Check sheet for the modelled part. Datum: model origin and axes. Units: mm. A direction names the side the tool comes from. Give positions to 0.01 mm unless a question says otherwise; leave off trailing zeros. Order: outer loops, then holes, each group sorted by start corner. A loop starts at its lowest first (then second) coordinate and runs counter-clockwise, first axis right, second up. Notation, with made-up numbers: (85.5, 55) -> (102.5, 55) arc R25 ccw to (102.5, 87) -> close; hole circle Ø8 at (76.5, 62). An arc over 180 degrees is marked (long way). Write each question's results on one line, items separated by ' | '.
from build123d import *

# Parameters (mm, degrees)
EXTRUDE1_DEPTH      = 2.794
CUT_EXTRUDE1_DEPTH  = 6.588
SHELL2_T            = 1.016
BOSS_EXTRUDE1_DEPTH = 5.08
BOSS_EXTRUDE2_DEPTH = 0.381


with BuildPart() as part:
    # Sketch1 → Extrude1 (new body, symmetric)
    with BuildSketch(Plane.XY):
        with BuildLine():
            Line((-83.497972353, 1.642657809), (-75.199494217, 5.08))
            Line((-75.199494217, 5.08), (75.199494217, 5.08))
            Line((75.199494217, 5.08), (83.497972353, 1.642657809))
            ThreePointArc((83.497972353, 1.642657809), (84.595561211, 0), (83.497972353, -1.642657809))
            Line((83.497972353, -1.642657809), (75.199494217, -5.08))
            Line((75.199494217, -5.08), (-75.199494217, -5.08))
            Line((-75.199494217, -5.08), (-83.497972353, -1.642657809))
            ThreePointArc((-83.497972353, -1.642657809), (-84.595561211, 0), (-83.497972353, 1.642657809))
        make_face()
    extrude(amount=EXTRUDE1_DEPTH, both=True)

    # Sketch7 → Cut-Extrude1 (cut, through all)
    with BuildSketch(Plane.XY.offset(-2.794)):
        with BuildLine():
            Line((-69.101561211, -1.905), (-68.593561211, -1.905))
            ThreePointArc((-68.593561211, -1.905), (-66.688561211, 0), (-68.593561211, 1.905))
            Line((-68.593561211, 1.905), (-69.101561211, 1.905))
            ThreePointArc((-69.101561211, 1.905), (-71.006561211, 0), (-69.101561211, -1.905))
        make_face()
        with BuildLine():
            Line((69.101561211, -1.905), (68.593561211, -1.905))
            ThreePointArc((68.593561211, -1.905), (66.688561211, 0), (68.593561211, 1.905))
            Line((68.593561211, 1.905), (69.101561211, 1.905))
            ThreePointArc((69.101561211, 1.905), (71.006561211, 0), (69.101561211, -1.905))
        make_face()
    extrude(amount=CUT_EXTRUDE1_DEPTH, mode=Mode.SUBTRACT)

    # Shell2 (no face opened: a closed hollow body)
    add(offset(amount=-SHELL2_T, mode=Mode.PRIVATE), mode=Mode.SUBTRACT)

    # Sketch16 → Boss-Extrude1 (add)
    with BuildSketch(Plane.XY):
        with BuildLine():
            Line((-68.593561211, 3.175), (-69.101561211, 3.175))
            ThreePointArc((-69.101561211, 3.175), (-72.276561211, 0), (-69.101561211, -3.175))
            Line((-69.101561211, -3.175), (-68.593561211, -3.175))
            ThreePointArc((-68.593561211, -3.175), (-65.418561211, 0), (-68.593561211, 3.175))
        make_face()
        with BuildLine():
            Line((-68.593561211, 1.905), (-69.101561211, 1.905))
            ThreePointArc((-69.101561211, 1.905), (-71.006561211, 0), (-69.101561211, -1.905))
            Line((-69.101561211, -1.905), (-68.593561211, -1.905))
            ThreePointArc((-68.593561211, -1.905), (-66.688561211, 0), (-68.593561211, 1.905))
        make_face(mode=Mode.SUBTRACT)
        with BuildLine():
            Line((69.101561211, -3.175), (68.593561211, -3.175))
            ThreePointArc((68.593561211, -3.175), (65.418561211, 0), (68.593561211, 3.175))
            Line((68.593561211, 3.175), (69.101561211, 3.175))
            ThreePointArc((69.101561211, 3.175), (72.276561211, 0), (69.101561211, -3.175))
        make_face()
        with BuildLine():
            Line((69.101561211, -1.905), (68.593561211, -1.905))
            ThreePointArc((68.593561211, -1.905), (66.688561211, 0), (68.593561211, 1.905))
            Line((68.593561211, 1.905), (69.101561211, 1.905))
            ThreePointArc((69.101561211, 1.905), (71.006561211, 0), (69.101561211, -1.905))
        make_face(mode=Mode.SUBTRACT)
    extrude(amount=BOSS_EXTRUDE1_DEPTH)

    # Sketch15 → Boss-Extrude2 (add)
    with BuildSketch(Plane(origin=(52.759975214, 8.567310029, 2.794), x_dir=(-1, 0, 0), z_dir=(0, 0, 1))):
        Polygon((30.833634894, 6.909260745), (29.58586719, 6.909260745), (30.209751042, 10.080670326), (31.457518746, 10.080670326), align=None)
        with BuildLine():
            Line((26.098109724, 6.909260745), (27.818196276, 10.080670326))
            Line((27.818196276, 10.080670326), (29.325915585, 10.080670326))
            Line((29.325915585, 10.080670326), (29.121363503, 9.040863906))
            Line((29.121363503, 9.040863906), (28.076751324, 9.040863906))
            ThreePointArc((28.076751324, 9.040863906), (27.966243867, 9.027758301), (27.861867206, 8.989168567))
            ThreePointArc((27.861867206, 8.989168567), (27.110933968, 8.112530186), (27.194312424, 6.961251066))
            Line((27.194312424, 6.961251066), (27.220239704, 6.909260745))
            Line((27.220239704, 6.909260745), (26.098109724, 6.909260745))
        make_face()
        with BuildLine():
            Line((24.594796374, 10.080670326), (25.024818012, 6.909260745))
            Line((25.024818012, 6.909260745), (23.345351563, 6.909260745))
            Line((23.345351563, 6.909260745), (23.451009312, 6.961251066))
            ThreePointArc((23.451009312, 6.961251066), (24.013843502, 7.721578938), (23.720459983, 8.620915865))
            ThreePointArc((23.720459983, 8.620915865), (23.664057171, 8.668518488), (23.600928958, 8.706756109))
            ThreePointArc((23.600928958, 8.706756109), (23.03751713, 8.93797936), (22.445309842, 9.080062458))
            ThreePointArc((22.445309842, 9.080062458), (22.355999269, 9.127094259), (22.313587173, 9.218688925))
            ThreePointArc((22.313587173, 9.218688925), (22.320050836, 9.315750612), (22.359212571, 9.404796153))
            ThreePointArc((22.359212571, 9.404796153), (22.441078376, 9.50688825), (22.550436966, 9.578759697))
            ThreePointArc((22.550436966, 9.578759697), (22.912840286, 9.660745811), (23.278270345, 9.593524078))
            ThreePointArc((23.278270345, 9.593524078), (23.448349032, 9.45576593), (23.512332705, 9.246457171))
            Line((23.512332705, 9.246457171), (23.512332705, 9.040863906))
            Line((23.512332705, 9.040863906), (24.334844769, 9.040863906))
            ThreePointArc((24.334844769, 9.040863906), (24.341195101, 9.582833311), (24.126883485, 10.080670326))
            Line((24.126883485, 10.080670326), (24.594796374, 10.080670326))
        make_face()
        with BuildLine():
            Line((28.312104326, 8.261009091), (28.967949441, 8.261009091))
            Line((28.967949441, 8.261009091), (28.814535379, 7.481154276))
            Line((28.814535379, 7.481154276), (28.209554826, 7.481154276))
            ThreePointArc((28.209554826, 7.481154276), (28.006347959, 7.565325317), (27.922176918, 7.768532184))
            Line((27.922176918, 7.768532184), (27.922176918, 7.871081684))
            ThreePointArc((27.922176918, 7.871081684), (28.036384012, 8.146801998), (28.312104326, 8.261009091))
        make_face()
        Polygon((25.790573757, 8.16352724), (25.706860528, 8.780912301), (26.125426672, 8.780912301), align=None)
        Polygon((25.530622152, 10.080670326), (26.830380177, 10.080670326), (26.576596915, 9.612757437), (25.594067968, 9.612757437), align=None)
        with BuildLine():
            Line((21.446019985, 6.986900983), (21.527856602, 6.905064366))
            Line((21.527856602, 6.905064366), (20.072127614, 6.905064366))
            ThreePointArc((20.072127614, 6.905064366), (21.073440916, 8.351729074), (20.74751262, 10.080670326))
            Line((20.74751262, 10.080670326), (21.839309361, 10.080670326))
            ThreePointArc((21.839309361, 10.080670326), (21.359771514, 9.203641008), (21.828371735, 8.320719265))
            ThreePointArc((21.828371735, 8.320719265), (21.970498458, 8.242561464), (22.123897961, 8.189861942))
            Line((22.123897961, 8.189861942), (22.959965448, 7.98084507))
            ThreePointArc((22.959965448, 7.98084507), (23.09929103, 7.88260745), (23.136218517, 7.716178461))
            ThreePointArc((23.136218517, 7.716178461), (23.063353728, 7.552354455), (22.917107557, 7.44862577))
            ThreePointArc((22.917107557, 7.44862577), (22.408346515, 7.486786133), (22.100511774, 7.893642107))
            Line((22.100511774, 7.893642107), (21.268666638, 7.893642107))
            ThreePointArc((21.268666638, 7.893642107), (21.219023851, 7.413217054), (21.446019985, 6.986900983))
        make_face()
        with BuildLine():
            Line((18.096006249, 6.909260745), (16.640277261, 6.909260745))
            ThreePointArc((16.640277261, 6.909260745), (17.684029363, 8.338941307), (17.368141755, 10.080670326))
            Line((17.368141755, 10.080670326), (18.66789978, 10.080670326))
            ThreePointArc((18.66789978, 10.080670326), (18.288993246, 9.583465168), (18.096006249, 8.988873585))
            Line((18.096006249, 8.988873585), (18.927851385, 8.988873585))
            ThreePointArc((18.927851385, 8.988873585), (19.124730401, 9.376543005), (19.462251482, 9.650638693))
            ThreePointArc((19.462251482, 9.650638693), (20.018996521, 9.643076799), (20.333746509, 9.183778785))
            ThreePointArc((20.333746509, 9.183778785), (20.297634521, 8.424922889), (20.010357156, 7.72161779))
            ThreePointArc((20.010357156, 7.72161779), (19.734264238, 7.404457918), (19.340648899, 7.256523307))
            ThreePointArc((19.340648899, 7.256523307), (18.807293319, 7.48101259), (18.719890101, 8.053047807))
            Line((18.719890101, 8.053047807), (17.784064323, 8.053047807))
            ThreePointArc((17.784064323, 8.053047807), (17.822649734, 7.449140035), (18.096006249, 6.909260745))
        make_face()
        with BuildLine():
            Line((15.807268249, 7.427425154), (15.715290544, 7.427425154))
            ThreePointArc((15.715290544, 7.427425154), (15.394442736, 7.543776842), (15.22275385, 7.838741175))
            ThreePointArc((15.22275385, 7.838741175), (15.210743896, 8.452467568), (15.392018164, 9.038934928))
            ThreePointArc((15.392018164, 9.038934928), (15.644599766, 9.361161911), (16.00483435, 9.555735132))
            ThreePointArc((16.00483435, 9.555735132), (16.126082831, 9.577672377), (16.249203287, 9.582549899))
            ThreePointArc((16.249203287, 9.582549899), (16.671437038, 9.390945472), (16.831737964, 8.95586248))
            ThreePointArc((16.831737964, 8.95586248), (16.709931987, 8.31539524), (16.410014233, 7.736530556))
            ThreePointArc((16.410014233, 7.736530556), (16.145960171, 7.509207095), (15.807268249, 7.427425154))
        make_face()
    extrude(amount=BOSS_EXTRUDE2_DEPTH)


solid = part.part
1. Material ranges on probe 1 along X at (y, z) = (0, 4); probe 2 along Y at (x, z) = (26.5, 0.5); probe 3 along Z at (x, y) = (-74.5, 2.75), recorded low to high. Write a range as from..to.
Verdict:
probe 1: x = -72.28..-71.01, -66.69..-65.42, 65.42..66.69, 71.01..72.28 | probe 2: y = -5.08..-4.06, 4.06..5.08 | probe 3: z = -2.79..-1.78, 1.78..2.79
2. Access from +Z, -Z, +X, -X, +Y, -Y to the whole of each face (thin tool, end or side, straight path). Record for faces 4 (the cylindrical face through (-72.276, 0.07, 3.921)), 5 (the flat face through (31.3, 0.4, 3.175)), 6 (the flat face through (78.997, 2.408, 0.025)).
Verdict:
face 4: +Z, -X | face 5: +Z, +Y, -Y | face 6: none
3. Gauge pin test, flat ends, axial feed: pin 1 Ø5 at (x, y) = (-20, -2.5) entering from +Z; pin 2 Ø0.8 at (x, y) = (37, 0) entering from +Z (3 decimals); pin 3 Ø3 at (y, z) = (2.5, 2) entering from +X. Record the tip position at first contact, or that the pin passes through.
Verdict:
pin 1: stops at z = 2.79 | pin 2: stops at z = 3.175 | pin 3: stops at x = 84.29
4. Section check A-A on x = -37. Record the cut outline in (y, z).
Verdict:
outline: (-5.08, -2.79) -> (5.08, -2.79) -> (5.08, 2.79) -> (-5.08, 2.79) -> close; hole (-4.06, -1.78) -> (4.06, -1.78) -> (4.06, 1.78) -> (-4.06, 1.78) -> close
5. Mould release check, pull along Z, two halves, no side actions. Record for faces 1 (the flat face through (-68.9, 2.2, 5.08)), 2 (the flat face through (1, 0, 1.778)), 3 (the cylindrical face through (84.595, 0.029, 0.039)): +Z half, -Z half, draft (parallel to the pull), parting line (faces both ways), or undercut.
Verdict:
face 1: +Z half | face 2: undercut | face 3: draft
